Can you work these out from the drawing? Everything is in mm from the part's minimum corner. A direction names the side the tool comes from. Round coordinates to 2 decimals unless told otherwise and drop trailing zeros. Write each loop counter-clockwise with the first axis right and the second up, starting at its lowest first coordinate (ties: lowest second). Pieces come first, ordered by that corner, then holes. Notation, with made-up numbers: (-37.5, 78.5) -> (-17.5, 78.5) arc R16 ccw to (-17.5, 83.5) -> close; hole circle Ø9 at (65.25, 54). An arc over 180 degrees is marked (long way). Answer as CSV lines item,"result".
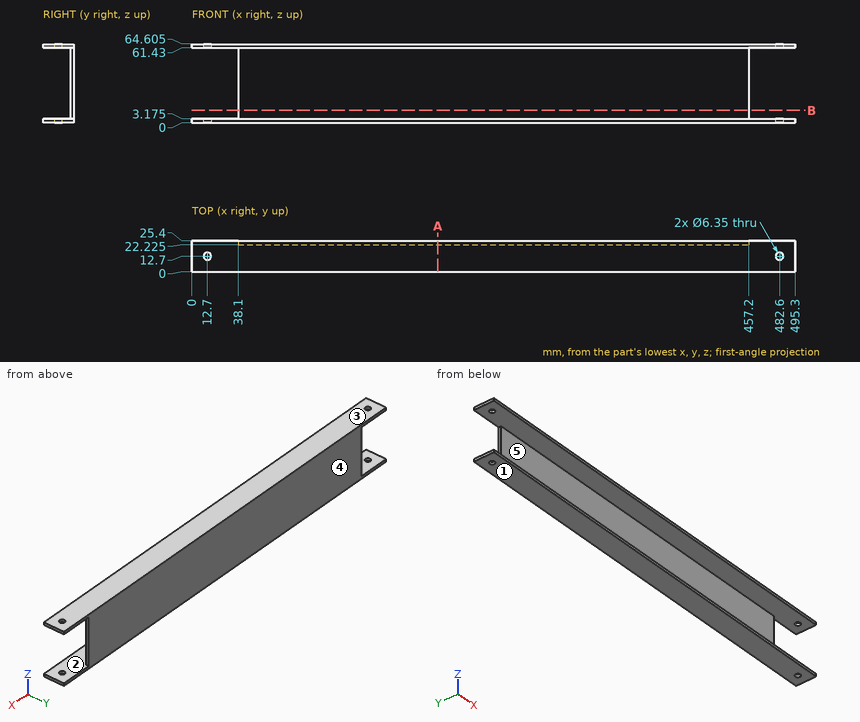
Item 1: Suppose I cut it at B-B, the plane z = 10. List the corners of the cut face in (x, y) for me (3 decimals).
Results found:
outline,"(38.1, 22.225) -> (457.2, 22.225) -> (457.2, 25.4) -> (38.1, 25.4) -> close"
Item 2: If we mould it in two halves opening along Z, with no side actions, what happens to the marked faces 1, 2 and 3? For each: pulls with the +Z half, pulls with the -Z half, needs draft (parallel to the pull), parting line crosses it, or undercut.
Results found:
face 1,"pulls with the -Z half"
face 2,"undercut"
face 3,"pulls with the +Z half"
Item 3: For the marked faces 4 and 5, which set-ups out of +Z, -Z, +X, -X, +Y, -Y let a thin tool reach every point of the face, with its end or its side?
Results found:
face 4,"+Z, -Z, +X, -X, +Y"
face 5,"+X, -X, -Y"
Item 4: Will these pins go through, and if not, where does the flat tip stop? pin 1 (4 mm diameter, centred on x = 12.7, y = 12.7, fed in from -Z); pin 2 (17.5 mm diameter, centred on x = 163, z = 25.5, fed in from -Y) (3 decimals); pin 3 (3.5 mm diameter, centred on y = 23.5, z = 29, fed in from -X); pin 4 (2.5 mm diameter, centred on y = 23, z = 45, fed in from +X).
Results found:
pin 1,"passes through"
pin 2,"stops at y = 22.225"
pin 3,"stops at x = 38.1"
pin 4,"stops at x = 457.2"
Item 5: I need wall thicknesses on L1, parallel to Z at x = 470, y = 15.5 (3 decimals); L2, parallel to Y at x = 482.6, z = 62.8 (3 decimals); L3, parallel to Y at x = 12, z = 63. Which ranges of each line are inside material? Lowest first, please.
Results found:
L1,"z = 0 to 3.175, 61.43 to 64.605"
L2,"y = 0 to 9.525, 15.875 to 25.4"
L3,"y = 0 to 9.6, 15.8 to 25.4"
Item 6: Suppose I cut it at A-A, the plane x = 202. List the corners of the cut face in (y, z) for me (3 decimals), then the cut area to 3 significant figures.
Results found:
outline,"(0, 0) -> (25.4, 0) -> (25.4, 64.605) -> (0, 64.605) -> (0, 61.43) -> (22.225, 61.43) -> (22.225, 3.175) -> (0, 3.175) -> close"
area,"346 mm²"
